Part model, mm, in its own coordinate system. A direction names the side the tool comes from. Round coordinates to 2 decimals unless told otherwise and drop trailing zeros. Loops run counter-clockwise (first coordinate to the right, second up) from the corner with the lowest first, then second, coordinate; pieces in that order, holes last. Notation, with made-up numbers: (-32.5, -31) - (-8.5, -31) arc R17 ccw to (-8.5, -18) - close; hole circle Ø11 at (8, 42). An arc over 180 degrees is marked (long way). Put each result on its own line as item: value.
from build123d import *

# Parameters (mm, degrees)
BOSS_EXTRUDE1_DEPTH = 6.35
CUT_EXTRUDE1_DEPTH  = 6.35


with BuildPart() as part:
    # Sketch1 → Boss-Extrude1 (new body)
    with BuildSketch(Plane(origin=(0, 0, 0), x_dir=(0, 0, -1), z_dir=(1, 0, 0))):
        Polygon((44.45, 0), (57.15, 0), (57.15, 6.35), (69.85, 6.35), (69.85, 0), (88.9, 0), (88.9, 6.35), (101.6, 6.35), (101.6, 19.05), (95.25, 19.05), (95.25, 39.37), (101.6, 39.37), (101.6, 49.53), (95.25, 49.53), (95.25, 69.85), (101.6, 69.85), (101.6, 82.55), (95.25, 82.55), (95.25, 88.9), (6.35, 88.9), (6.35, 82.55), (0, 82.55), (0, 69.85), (6.35, 69.85), (6.35, 49.53), (0, 49.53), (0, 39.37), (6.35, 39.37), (6.35, 19.05), (0, 19.05), (0, 6.35), (12.7, 6.35), (12.7, 0), (31.75, 0), (31.75, 6.35), (44.45, 6.35), align=None)
    extrude(amount=BOSS_EXTRUDE1_DEPTH)

    # Sketch2 → Cut-Extrude1 (cut)
    with BuildSketch(Plane(origin=(6.35, 0, 0), x_dir=(0, 0, -1), z_dir=(1, 0, 0))):
        Polygon((44.45, 47.625), (22.452954744, 60.325), (22.452954744, 34.925), align=None)
        Polygon((50.8, 53.975), (63.5, 75.972045256), (38.1, 75.972045256), align=None)
        Polygon((57.15, 47.625), (79.147045256, 34.925), (79.147045256, 60.325), align=None)
        Polygon((50.8, 41.275), (38.1, 19.277954744), (63.5, 19.277954744), align=None)
    extrude(amount=-CUT_EXTRUDE1_DEPTH, mode=Mode.SUBTRACT)


solid = part.part
1. Pin check, flat tips, straight feed: P1, Ø1, axis at x = 4, z = -44.5, coming from the -Y side; P2, Ø3, axis at x = 1.5, z = -65, coming from the -Y side; P3, Ø3, axis at x = 4, y = 24.5, coming from the +Z side; P4, Ø3, axis at x = 2.5, y = 60, coming from the -Z side. Stop position of each tip, or through.
A:
P1: stops at y = 0
P2: stops at y = 6.35
P3: stops at z = -6.35
P4: stops at z = -95.25
2. Band-saw the part on D-D (z = -53). List the corners of the cut face in (x, y).
A:
outline: (0, 0) - (6.35, 0) - (6.35, 19.28) - (0, 19.28) - close; (0, 37.46) - (6.35, 37.46) - (6.35, 57.79) - (0, 57.79) - close; (0, 75.97) - (6.35, 75.97) - (6.35, 88.9) - (0, 88.9) - close
3. Two-plate mould, pull along Z, no slides. Class faces 1 (the flat face through (3, 6.35, -38)), 2 (the flat face through (3, 60, -6.35)), 3 (the flat face through (3, 88.9, -51)), 4 (the flat face through (3.22, 64.82, -57.06)): pulls with the +Z half, pulls with the -Z half, needs draft (parallel to the pull), parting line crosses it, or undercut.
A:
face 1: undercut
face 2: pulls with the +Z half
face 3: needs draft
face 4: undercut
4. Band-saw the part on A-A (z = -78). List the corners of the cut face in (x, y), plus the area to 3 significant figures.
A:
outline: (0, 0) - (6.35, 0) - (6.35, 35.59) - (0, 35.59) - close; (0, 59.66) - (6.35, 59.66) - (6.35, 88.9) - (0, 88.9) - close
area: 412 mm²
5. Probe line 1 along Z through (x, y) = (1.5, 48); line 2 along Y through (x, z) = (1.5, -50); line 3 along Z through (x, y) = (3.5, 39). List the from-to ranges inside material, lowest first. Write a range as [from, to].
A:
line 1: z = [-101.6, -79.15], [-57.8, -43.8], [-22.45, 0]
line 2: y = [0, 19.28], [39.89, 55.36], [75.97, 88.9]
line 3: z = [-95.25, -79.15], [-72.09, -52.11], [-49.49, -29.51], [-22.45, -6.35]
6. Tool access for faces 5 (the flat face through (3.22, 65.13, -44.36)), 6 (the flat face through (3, 19.05, -98)), 7 (the flat face through (3, 86, -6.35)), 8 (the flat face through (3, 3, -12.7)): list every direction of +Z, -Z, +X, -X, +Y, -Y with a clear straight run to the whole face (end or side of a thin tool).
A:
face 5: +X, -X
face 6: -Z, +X, -X
face 7: +Z, +X, -X, +Y
face 8: +Z, +X, -X, -Y
7. Band-saw the part on C-C (y = 51). List the corners of the cut face in (x, z).
A:
outline: (0, -95.25) - (6.35, -95.25) - (6.35, -79.15) - (0, -79.15) - close; (0, -63) - (6.35, -63) - (6.35, -38.6) - (0, -38.6) - close; (0, -22.45) - (6.35, -22.45) - (6.35, -6.35) - (0, -6.35) - close
8. Band-saw the part on B-B (y = 30). List the corners of the cut face in (x, z).
A:
outline: (0, -95.25) - (6.35, -95.25) - (6.35, -57.31) - (0, -57.31) - close; (0, -44.29) - (6.35, -44.29) - (6.35, -6.35) - (0, -6.35) - close
